```python
from build123d import *

# Parameters (mm, degrees)
F0_R     = 46.75
F1_DEPTH = 3
F2_R     = 43.6
F3_DEPTH = 25.4
F4_R     = 37.1
F4_R_2   = 36.1
F4_R_3   = 18.5
F4_R_4   = 17.5
F5_DEPTH = 1
F7_DEPTH = 25.4
F8_R     = 6.375059
F9_DEPTH = 3.001


with BuildPart() as f1:
    # F0 (on Top) → F1 (new body)
    with BuildSketch(Plane.XY):
        Circle(F0_R)
    extrude(amount=F1_DEPTH)

    # F2 (on face) → F3 (join)
    with BuildSketch(Plane.XY.offset(3)):
        Circle(F2_R)
    extrude(amount=F3_DEPTH)

    # F4 (on face) → F5 (cut)
    with BuildSketch(Plane(origin=(0, 0, 0), x_dir=(1, 0, 0), z_dir=(0, 0, -1))):
        Circle(F4_R)
        Circle(F4_R_2, mode=Mode.SUBTRACT)
        Circle(F4_R_3)
        Circle(F4_R_4, mode=Mode.SUBTRACT)
    extrude(amount=-F5_DEPTH, mode=Mode.SUBTRACT)

    # F6 (on face) → F7 (cut, through all)
    with BuildSketch(Plane.XY.offset(28.4)):
        with BuildLine():
            Line((-1.884867, -40.050467), (-1.884867, -1.939485))
            Line((-1.884867, -1.939485), (-40.047859, -1.939485))
            ThreePointArc((-40.047859, -1.939485), (-28.331963, -28.370627), (-1.884867, -40.050467))
        make_face()
        with BuildLine():
            Line((-40.039012, 2.114258), (-1.884867, 2.114258))
            Line((-1.884867, 2.114258), (-1.884867, 40.050467))
            ThreePointArc((-1.884867, 40.050467), (-28.269982, 28.432388), (-40.039012, 2.114258))
        make_face()
        with BuildLine():
            Line((2.048553, 40.042428), (2.048553, 2.114258))
            Line((2.048553, 2.114258), (40.039012, 2.114258))
            ThreePointArc((40.039012, 2.114258), (28.32803, 28.374554), (2.048553, 40.042428))
        make_face()
        with BuildLine():
            Line((40.047859, -1.939485), (2.048553, -1.939485))
            Line((2.048553, -1.939485), (2.048553, -40.042428))
            ThreePointArc((2.048553, -40.042428), (28.389884, -28.312666), (40.047859, -1.939485))
        make_face()
    extrude(amount=-F7_DEPTH, mode=Mode.SUBTRACT)

    # F8 (on face) → F9 (cut, through all)
    with BuildSketch(Plane.XY.offset(3)):
        with Locations((-16.523598, 16.523598)):
            Circle(F8_R)
        with Locations((16.523598, 16.523598)):
            Circle(F8_R)
        with Locations((16.523598, -16.523598)):
            Circle(F8_R)
        with Locations((-16.523598, -16.523598)):
            Circle(F8_R)
    extrude(amount=-F9_DEPTH, mode=Mode.SUBTRACT)


solid = f1.part
```
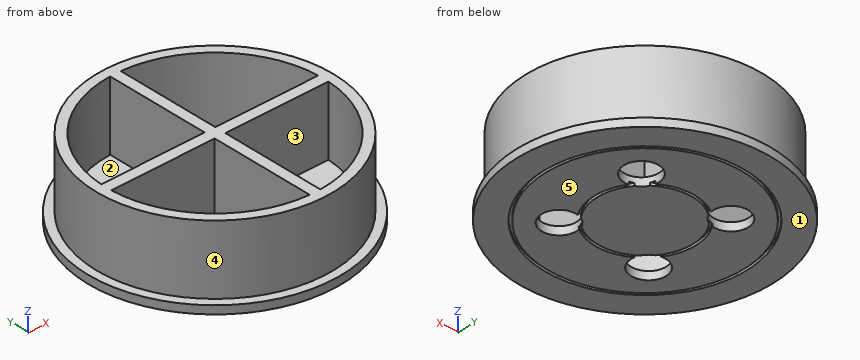
Source: CAD feature listing. Evaluate the final solid. Frame: model axes, mm. Face numbers are marked on the shaded views. A direction names the side the tool comes from. Coordinates: 2 decimals unless noted, no trailing zeros. Write each loop counter-clockwise with the first axis right and the second up, starting at its lowest first coordinate (ties: lowest second). Pieces come first, ordered by that corner, then holes. Notation, with made-up numbers: (61.25, 56.25) -> (72.25, 56.25) arc R18 ccw to (72.25, 89.25) -> close; hole circle Ø11 at (26.5, 79). An arc over 180 degrees is marked (long way). Return JSON: item names as keys, results as strings. Group by question number.
1) Set-up query: the marked faces 1 and 2. Return all of +Z, -Z, +X, -X, +Y, -Y with unobstructed straight access to the full face (end or side cutting, diameter ignored); none if empty.
2) Section query A-A, the plane z = 22.25. Return loops of the section in (x, y).
3) Ray query, line 1 along Y through (x, z) = (-6.5, 19); line 2 along Y through (x, z) = (-16, 3.5); line 3 along X through (y, z) = (25.5, 21.5). Return the intervals inside material, ascending.
4) Section query B-B, the plane y = 0. Return loops of the section in (x, z), plus the area to 3 significant figures.
5) Contact query for flat-ended pins moving along their axis: P1, Ø10, axis at x = -20.5, z = 4.5, coming from the +Y side; P2, Ø3, axis at y = -35, z = 21, coming from the +X side; P3, Ø6, axis at x = -24.5, z = 4, coming from the -Y side. Output: stop coordinate, or through.
6) Mould query, pull axis Y, two halves, no side actions, for the marked faces 3, 4 and 5. Classes: +Y half, -Y half, draft (parallel to the pull), parting line (faces both ways), or undercut.
From the geometry:
{
 "1": {"face 1": "-Z, +X, -X, +Y, -Y", "face 2": "+Z"},
 "2": {"outline": "circle Ø87.2 at (0, 0); hole (-40.05, -1.94) arc R40.09 ccw to (-1.88, -40.05) -> (-1.88, -1.94) -> close; hole (-40.04, 2.11) -> (-1.88, 2.11) -> (-1.88, 40.05) arc R40.09 ccw to start; hole (2.05, -40.04) arc R40.09 ccw to (40.05, -1.94) -> (2.05, -1.94) -> close; hole (2.05, 2.11) -> (40.04, 2.11) arc R40.09 ccw to (2.05, 40.04) -> close"},
 "3": {"line 1": "-43.11 to -39.56, -1.94 to 2.11, 39.56 to 43.11", "line 2": "-40.56 to -36.76, -1.94 to 2.11, 36.76 to 40.56", "line 3": "-35.37 to -30.94, -1.88 to 2.05, 30.94 to 35.37"},
 "4": {"outline": "(-46.75, 0) -> (-37.1, 0) -> (-37.1, 1) -> (-36.1, 1) -> (-36.1, 0) -> (-18.5, 0) -> (-18.5, 1) -> (-17.5, 1) -> (-17.5, 0) -> (17.5, 0) -> (17.5, 1) -> (18.5, 1) -> (18.5, 0) -> (36.1, 0) -> (36.1, 1) -> (37.1, 1) -> (37.1, 0) -> (46.75, 0) -> (46.75, 3) -> (43.6, 3) -> (43.6, 28.4) -> (-43.6, 28.4) -> (-43.6, 3) -> (-46.75, 3) -> close", "area": "2,490 mm²"},
 "5": {"P1": "y = 44.02", "P2": "x = 27.91", "P3": "y = -41.42"},
 "6": {"face 3": "undercut", "face 4": "parting line", "face 5": "draft"}
}
